Verification items for the finished model (mm, model axes). Face numbers are marked on the shaded views. A direction names the side the tool comes from. Give positions to 0.01 mm unless a question says otherwise; leave off trailing zeros. Write each loop counter-clockwise with the first axis right and the second up, starting at its lowest first coordinate (ties: lowest second). Pieces come first, ordered by that corner, then holes. Notation, with made-up numbers: (62, -33) - (87, -33) arc R19 cw to (87, -16) - close; hole circle Ø4 at (54.25, 39). An arc over 180 degrees is marked (long way). Put each result on its own line as item: value.
from build123d import *

# Parameters (mm, degrees)
SKETCH1_R           = 95
BOSS_EXTRUDE1_DEPTH = 20
SKETCH2_R           = 45
BOSS_EXTRUDE2_DEPTH = 55
SKETCH4_R           = 22.5
CUT_EXTRUDE1_DEPTH  = 75
SKETCH5_R           = 6
CUT_EXTRUDE2_DEPTH  = 20
SKETCH6_W           = 14
SKETCH6_H           = 4
CUT_EXTRUDE3_DEPTH  = 154.866825534
FILLET1_R           = 3


with BuildPart() as part:
    # Sketch1 → Boss-Extrude1 (new body)
    with BuildSketch(Plane(origin=(0, 0, 0), x_dir=(0, 0, -1), z_dir=(1, 0, 0))):
        Circle(SKETCH1_R)
    extrude(amount=-BOSS_EXTRUDE1_DEPTH)

    # Sketch2 → Boss-Extrude2 (add)
    with BuildSketch(Plane.ZY.offset(20)):
        Circle(SKETCH2_R)
    extrude(amount=BOSS_EXTRUDE2_DEPTH)

    # Sketch4 → Cut-Extrude1 (cut)
    with BuildSketch(Plane(origin=(0, 0, 0), x_dir=(0, 0, -1), z_dir=(1, 0, 0))):
        Circle(SKETCH4_R)
    extrude(amount=-CUT_EXTRUDE1_DEPTH, mode=Mode.SUBTRACT)

    # Sketch5 → Cut-Extrude2 (cut)
    with BuildSketch(Plane(origin=(0, 0, 0), x_dir=(0, 0, -1), z_dir=(1, 0, 0))):
        with Locations((0, 70)):
            Circle(SKETCH5_R)
        with Locations((70, 0)):
            Circle(SKETCH5_R)
        with Locations((0, -70)):
            Circle(SKETCH5_R)
        with Locations((-70, 0)):
            Circle(SKETCH5_R)
    extrude(amount=-CUT_EXTRUDE2_DEPTH, mode=Mode.SUBTRACT)

    # Sketch6 → Cut-Extrude3 (cut, through all)
    with BuildSketch(Plane(origin=(0, 0, 0), x_dir=(0, 0, -1), z_dir=(1, 0, 0))):
        with Locations((0, 23.38340478)):
            Rectangle(SKETCH6_W, SKETCH6_H)
    extrude(amount=-CUT_EXTRUDE3_DEPTH, mode=Mode.SUBTRACT)

    # Fillet1
    fillet1_edges = [part.edges().sort_by_distance(p)[0] for p in [
        (-20, 0, 95),
        (-20, 0, -45),
        (-75, 0, -45),
    ]]
    fillet(fillet1_edges, radius=FILLET1_R)


solid = part.part
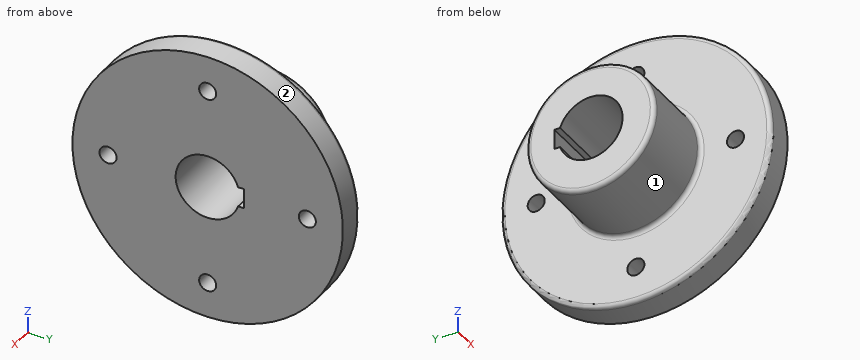
Q1. Scan lines: line 1 along X through (y, z) = (64.5, 21.5); line 2 along Z through (x, y) = (-62, -1.5) (3 decimals); line 3 along Y through (x, z) = (-66, -11). Record each from-to range of solid material in increasing order.
Answers follow:
line 1: x = -20 to 0
line 2: z = -44.975 to -22.45, 22.45 to 44.975
line 3: y = -43.63 to -19.63, 19.63 to 43.63
Q2. Go/stop test with flat-tipped pins: pin 1 Ø11 at (y, z) = (-70, 0) entering from +X; pin 2 Ø3 at (x, y) = (-44, -2.5) entering from -Z; pin 3 Ø10 at (x, z) = (-38, -46) entering from +Y; pin 4 Ø4 at (x, z) = (-43.5, 1) entering from -Y. Record where each tip stops, or that it passes through.
Answers follow:
pin 1: passes through
pin 2: stops at z = -44.99
pin 3: stops at y = 18.55
pin 4: stops at y = -45
Q3. Section check A-A, the plane y = 0. Record the cut outline in (x, z), plus the area to 3 significant figures.
Answers follow:
outline: (-75, -42) arc R3 ccw to (-72, -45) - (-23, -45) arc R3 cw to (-20, -48) - (-20, -64) - (0, -64) - (0, -22.5) - (-75, -22.5) - close; (-75, 22.5) - (0, 22.5) - (0, 64) - (-20, 64) - (-20, 48) arc R3 cw to (-23, 45) - (-72, 45) arc R3 ccw to (-75, 42) - close; (-20, -92) arc R3 ccw to (-17, -95) - (0, -95) - (0, -76) - (-20, -76) - close; (-20, 76) - (0, 76) - (0, 95) - (-17, 95) arc R3 ccw to (-20, 92) - close
area: 4,890 mm2
Q4. Section check B-B, the plane x = -67. Record the cut outline in (y, z), plus the area to 3 significant figures.
Answers follow:
outline: circle Ø90 at (0, 0); hole (21.38, -7) - (25.38, -7) - (25.38, 7) - (21.38, 7) arc R22.5 ccw (long way) to start
area: 4,730 mm2
Q5. Set-up check for the marked faces 1 and 2: record each of +Z, -Z, +X, -X, +Y, -Y from which the full face is reachable in a straight line by a thin tool's end or side.
Answers follow:
face 1: -X
face 2: +X, -X
